For this review, take the finished solid that the model builds, in its own axes (mm). A direction names the side the tool comes from. Give positions to 0.01 mm unless a question says otherwise; leave off trailing zeros. Order: outer loops, then holes, each group sorted by start corner. A loop starts at its lowest first (then second) coordinate and runs counter-clockwise, first axis right, second up. Notation, with made-up numbers: (37.25, -7) -> (72.25, -7) arc R14 ccw to (72.25, 0) -> close; hole circle Ø5 at (30, 7). An arc over 180 degrees is marked (long way). One line per item, written item: value. Start each with the question number.
from build123d import *

# Parameters (mm, degrees)
SKETCH_1_R      = 21
SKETCH_1_R_2    = 12.5
EXTRUDE_1_DEPTH = 4.5
SKETCH_2_R      = 3.05
EXTRUDE_3_DEPTH = 3.5
SKETCH_3_R      = 21
SKETCH_3_R_2    = 14.5
EXTRUDE_4_DEPTH = 0.2
SKETCH_5_R      = 21
SKETCH_5_R_2    = 14.5
EXTRUDE_8_DEPTH = 0.2
SKETCH_6_R      = 21
SKETCH_6_R_2    = 12.5
EXTRUDE_9_DEPTH = 4.5


with BuildPart() as part:
    # Sketch 1 → Extrude 1 (new body)
    with BuildSketch(Plane(origin=(0, 0, 0), x_dir=(1, 0, 0), z_dir=(0, 1, 0))):
        with Locations(Location((0, 0, 0), (0, 0, 270))):
            Circle(SKETCH_1_R)
        with Locations(Location((0, 0, 0), (0, 0, 270))):
            Circle(SKETCH_1_R_2, mode=Mode.SUBTRACT)
    extrude(amount=EXTRUDE_1_DEPTH)

    # Sketch 2 → Extrude 3 (add)
    with BuildSketch(Plane(origin=(0, 4.5, 0), x_dir=(1, 0, 0), z_dir=(0, 1, 0))):
        with Locations(Location((0, 16.75, 0), (0, 0, 270))):
            Circle(SKETCH_2_R)
        with Locations(Location((6.050797909, 15.618909843, 0), (0, 0, 270))):
            Circle(SKETCH_2_R)
        with Locations(Location((11.284402031, 12.378399363, 0), (0, 0, 270))):
            Circle(SKETCH_2_R)
        with Locations(Location((14.99398513, 7.466117459, 0), (0, 0, 270))):
            Circle(SKETCH_2_R)
        with Locations(Location((16.678547453, 1.545495021, 0), (0, 0, 270))):
            Circle(SKETCH_2_R)
        with Locations(Location((16.110579523, -4.583855084, 0), (0, 0, 270))):
            Circle(SKETCH_2_R)
        with Locations(Location((13.366788557, -10.094130159, 0), (0, 0, 270))):
            Circle(SKETCH_2_R)
        with Locations(Location((8.817738728, -14.241137023, 0), (0, 0, 270))):
            Circle(SKETCH_2_R)
        with Locations(Location((3.077804423, -16.46479942, 0), (0, 0, 270))):
            Circle(SKETCH_2_R)
        with Locations(Location((-3.077804423, -16.46479942, 0), (0, 0, 270))):
            Circle(SKETCH_2_R)
        with Locations(Location((-8.817738728, -14.241137023, 0), (0, 0, 270))):
            Circle(SKETCH_2_R)
        with Locations(Location((-13.366788557, -10.094130159, 0), (0, 0, 270))):
            Circle(SKETCH_2_R)
        with Locations(Location((-16.110579523, -4.583855084, 0), (0, 0, 270))):
            Circle(SKETCH_2_R)
        with Locations(Location((-16.678547453, 1.545495021, 0), (0, 0, 270))):
            Circle(SKETCH_2_R)
        with Locations(Location((-14.99398513, 7.466117459, 0), (0, 0, 270))):
            Circle(SKETCH_2_R)
        with Locations(Location((-11.284402031, 12.378399363, 0), (0, 0, 270))):
            Circle(SKETCH_2_R)
        with Locations(Location((-6.050797909, 15.618909843, 0), (0, 0, 270))):
            Circle(SKETCH_2_R)
    extrude(amount=EXTRUDE_3_DEPTH)

    # Sketch 5 → Extrude 8 (add)
    with BuildSketch(Plane(origin=(0, 4.5, 0), x_dir=(1, 0, 0), z_dir=(0, 1, 0))):
        with Locations(Location((0, 0, 0), (0, 0, 270))):
            Circle(SKETCH_5_R)
        with Locations(Location((0, 0, 0), (0, 0, 270))):
            Circle(SKETCH_5_R_2, mode=Mode.SUBTRACT)
    extrude(amount=EXTRUDE_8_DEPTH)



with BuildPart() as body_2:
    # Sketch 3 → Extrude 4 (new body)
    with BuildSketch(Plane(origin=(0, 6.5, 0), x_dir=(1, 0, 0), z_dir=(0, 1, 0))):
        with Locations(Location((0, 0, 0), (0, 0, 270))):
            Circle(SKETCH_3_R)
        with Locations(Location((0, 0, 0), (0, 0, 270))):
            Circle(SKETCH_3_R_2, mode=Mode.SUBTRACT)
    extrude(amount=-EXTRUDE_4_DEPTH)


with BuildPart() as part_1:
    add(part.part)

    add(body_2.part)  # Extrude 9 merges body 2
    # Sketch 6 → Extrude 9 (add)
    with BuildSketch(Plane(origin=(0, 6.5, 0), x_dir=(1, 0, 0), z_dir=(0, 1, 0))):
        with Locations(Location((0, 0, 0), (0, 0, 270))):
            Circle(SKETCH_6_R)
        with Locations(Location((0, 0, 0), (0, 0, 270))):
            Circle(SKETCH_6_R_2, mode=Mode.SUBTRACT)
    extrude(amount=EXTRUDE_9_DEPTH)


solid = part_1.part
Q1. For faces 1 (the cylindrical face through (3.755, 2.218, 11.923)), 2 (the cylindrical face through (6.97, 5.49, -12.71)), list the 3-axis set-ups (+Z, -Z, +X, -X, +Y, -Y) from which the entire face can be reached by the end or side of a thin tool; tool diameter is ignored.
Q2. Take a section at D-D (y = 1). State the section outline as (x, z) points, and give its area (3 significant figures).
Q3. Take a section at C-C (z = 0). State the section outline as (x, y) points.
Q4. Take a section at B-B (x = -4). State the section outline as (y, z) points.
Q5. For line 1 along X through (y, z) = (2, 0); line 2 along Y through (x, z) = (-2, -13); line 3 along X through (y, z) = (10, 5.5), list the stretches that pass through material, from the lowest coordinate up.
Q6. For pin 1 Ø6 at (x, y) = (5, 6) entering from -Z; pin 2 Ø1.5 at (x, y) = (-10, 3.5) entering from +Z; pin 3 Ø4 at (x, y) = (8.5, 9.5) entering from +Z; pin 4 Ø5 at (x, z) = (-0.5, -9) entering from +Y, all flat-tipped, find the tip position at first contact; note any pin that passes through.
Q7. Take a section at A-A (y = 5.25). State how many separate pieces and enclosed holes the cut face has, and give its area (3 significant figures).
Answers below:
1. face 1: +Y, -Y
1. face 2: none
2. outline: circle Ø42 at (0, 0); hole circle Ø25 at (0, 0)
2. area: 895 mm²
3. outline: (-21, 0) -> (-12.5, 0) -> (-12.5, 4.5) -> (-14.05, 4.5) -> (-14.05, 6.5) -> (-12.5, 6.5) -> (-12.5, 11) -> (-21, 11) -> (-21, 6.3) -> (-19.31, 6.3) -> (-19.31, 4.7) -> (-21, 4.7) -> close; (12.5, 0) -> (21, 0) -> (21, 4.7) -> (19.31, 4.7) -> (19.31, 6.3) -> (21, 6.3) -> (21, 11) -> (12.5, 11) -> (12.5, 6.5) -> (14.05, 6.5) -> (14.05, 4.5) -> (12.5, 4.5) -> close
4. outline: (0, -20.62) -> (4.7, -20.62) -> (4.7, -17.88) -> (6.3, -17.88) -> (6.3, -20.62) -> (11, -20.62) -> (11, -11.84) -> (6.5, -11.84) -> (6.5, -13.36) -> (4.5, -13.36) -> (4.5, -11.84) -> (0, -11.84) -> close; (0, 11.84) -> (4.5, 11.84) -> (4.5, 13.56) -> (6.5, 13.56) -> (6.5, 11.84) -> (11, 11.84) -> (11, 20.62) -> (6.3, 20.62) -> (6.3, 19.37) -> (4.7, 19.37) -> (4.7, 20.62) -> (0, 20.62) -> close
5. line 1: x = -21 to -12.5, 12.5 to 21
5. line 2: y = 0 to 4.5, 6.5 to 11
5. line 3: x = -20.27 to -11.22, 11.22 to 20.27
6. pin 1: stops at z = -20.9
6. pin 2: stops at z = 18.85
6. pin 3: stops at z = 19.97
6. pin 4: passes through
7. separate pieces: 17
7. enclosed holes: 0
7. area: 497 mm²
